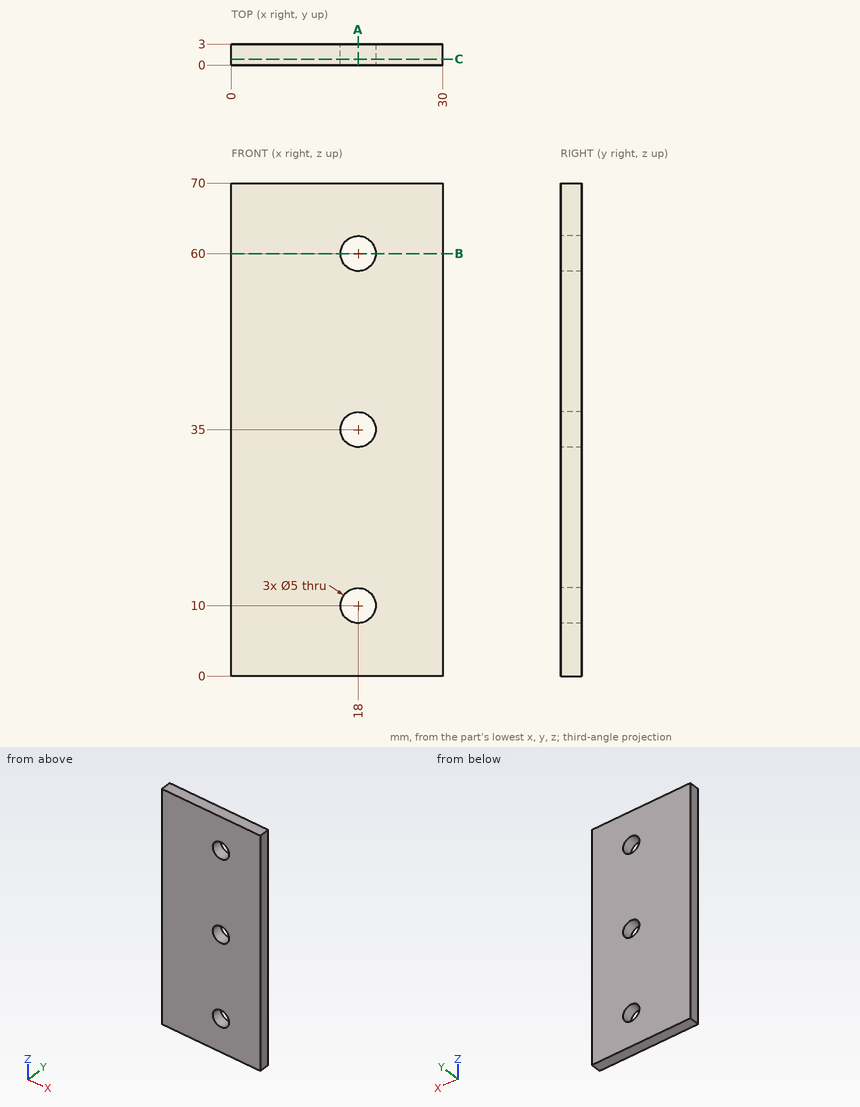
Can you work these out from the drawing? Everything is in mm from the part's minimum corner. Coordinates: 2 decimals unless noted, no trailing zeros. Write each loop counter-clockwise with the first axis right and the second up, starting at its lowest first coordinate (ties: lowest second). Pieces come first, ordered by that corner, then holes. Notation, with made-up numbers: (32.25, -40) - (74.25, -40) arc R26 ccw to (74.25, -17) - close; hole circle Ø3 at (68, 45.5). An arc over 180 degrees is marked (long way). Use a Markdown table: item, result.
Q1. Imagine slicing it at A-A (x = 18). List the corners of the cut face in (y, z) for me.
Geometry check:
| item | result |
|---|---|
| outline | (0, 0) - (3, 0) - (3, 7.5) - (0, 7.5) - close; (0, 12.5) - (3, 12.5) - (3, 32.5) - (0, 32.5) - close; (0, 37.5) - (3, 37.5) - (3, 57.5) - (0, 57.5) - close; (0, 62.5) - (3, 62.5) - (3, 70) - (0, 70) - close |
Q2. Please list where these lines run through material, in increasing order: L1, parallel to Z at x = 18, y = 1.6; L2, parallel to Z at x = 16, y = 2.05; L3, parallel to X at y = 1.2, z = 60.5.
Geometry check:
| item | result |
|---|---|
| L1 | z = 0 to 7.5, 12.5 to 32.5, 37.5 to 57.5, 62.5 to 70 |
| L2 | z = 0 to 8.5, 11.5 to 33.5, 36.5 to 58.5, 61.5 to 70 |
| L3 | x = 0 to 15.55, 20.45 to 30 |
Q3. I'm going to push a flat-ended pin straight in: pin 1 Ø4 at (x, z) = (18, 10) entering from -Y. Where does the tip first touch, or does it pass through?
Geometry check:
| item | result |
|---|---|
| pin 1 | passes through |
Q4. Imagine slicing it at C-C (y = 0.85). List the corners of the cut face in (x, z) for me.
Geometry check:
| item | result |
|---|---|
| outline | (0, 0) - (30, 0) - (30, 70) - (0, 70) - close; hole circle Ø5 at (18, 10); hole circle Ø5 at (18, 35); hole circle Ø5 at (18, 60) |
Q5. Imagine slicing it at B-B (z = 60). List the corners of the cut face in (x, y) for me, and give its area (3 significant figures).
Geometry check:
| item | result |
|---|---|
| outline | (0, 0) - (15.5, 0) - (15.5, 3) - (0, 3) - close; (20.5, 0) - (30, 0) - (30, 3) - (20.5, 3) - close |
| area | 75.0 mm2 |
